from build123d import *

# Parameters (mm, degrees)
SKETCH1_W           = 800
SKETCH1_H           = 650
BOSS_EXTRUDE1_DEPTH = 200
SKETCH2_W           = 796
SKETCH2_H           = 646
CUT_EXTRUDE1_DEPTH  = 198
CUT_EXTRUDE3_REACH  = 802
SKETCH4_R           = 30


with BuildPart() as part:
    # Sketch1 → Boss-Extrude1 (new body)
    with BuildSketch(Plane(origin=(0, 0, 0), x_dir=(1, 0, 0), z_dir=(0, 1, 0))):
        with Locations((400, 325)):
            Rectangle(SKETCH1_W, SKETCH1_H)
    extrude(amount=BOSS_EXTRUDE1_DEPTH)

    # Sketch2 → Cut-Extrude1 (cut)
    with BuildSketch(Plane(origin=(0, 200, 0), x_dir=(1, 0, 0), z_dir=(0, 1, 0))):
        with Locations((400, 325)):
            Rectangle(SKETCH2_W, SKETCH2_H)
    extrude(amount=-CUT_EXTRUDE1_DEPTH, mode=Mode.SUBTRACT)

    # Sketch4 → Cut-Extrude3 (cut, up to next)
    with BuildSketch(Plane(origin=(800, 0, 0), x_dir=(0, 0, -1), z_dir=(1, 0, 0)), mode=Mode.PRIVATE) as cut_extrude3_sk1:
        with Locations((325, 40)):
            Circle(SKETCH4_R)
    cut_extrude3_tool1 = extrude(cut_extrude3_sk1.sketch, amount=-CUT_EXTRUDE3_REACH, mode=Mode.PRIVATE) & part.part
    add(cut_extrude3_tool1.solids().sort_by_distance((800, 40, -325))[0], mode=Mode.SUBTRACT)


solid = part.part
Verification items for the finished model (mm, model axes). A direction names the side the tool comes from. Give positions to 0.01 mm unless a question says otherwise; leave off trailing zeros. Order: outer loops, then holes, each group sorted by start corner. A loop starts at its lowest first (then second) coordinate and runs counter-clockwise, first axis right, second up. Notation, with made-up numbers: M 2.5,84.5 L 52.5,84.5 A23 cw 52.5,112.5 Z; hole C 13.5,-39 d10. An arc over 180 degrees is marked long. Use one line per item in the form item = value. Start each with the question number.
Q1. Scan lines: line 1 along Z through (x, y) = (521.5, 53); line 2 along Y through (x, z) = (799.3, -325); line 3 along X through (y, z) = (33.5, -289). Record each from-to range of solid material in increasing order. Write a range as [from, to].
Q2. Section check C-C (x = 444). Enter the section's corners in (y, z), then the cut area to 3 significant figures.
Q3. Section check B-B (z = -325). Enter the section's corners in (x, y), then the cut area to 3 significant figures.
Q4. Go/stop test with a flat-tipped pin: pin 1 Ø8 at (x, z) = (439.5, -473.5) entering from +Y. Record where the tip stops, or that it passes through.
Q5. Mould release check, pull along X, two halves, no side actions. Record for faces 1 (the flat face through (394, 102, -648)), 2 (the flat face through (0, 99, -320)), 3 (the cylindrical face through (799.01, 41.32, -295.03)), 4 (the flat face through (800, 99, -320)): +X half, -X half, draft (parallel to the pull), parting line (faces both ways), or undercut.
Q6. Section check A-A (y = 188). Enter the section's corners in (x, z).
Q7. Section check D-D (y = 40). Enter the section's corners in (x, z), then the cut area to 3 significant figures.
Q8. Access from +Z, -Z, +X, -X, +Y, -Y to the whole of each face (thin tool, end or side, straight path). Record for faces 5 (the flat face through (394, 0, -330)), 6 (the flat face through (394, 2, -330)).
Evaluation:
q1.line_1 = [-650, -648], [-2, 0]
q1.line_2 = [0, 10], [70, 200]
q1.line_3 = [0, 2], [798, 800]
q2.outline = M 0,-650 L 200,-650 L 200,-648 L 2,-648 L 2,-2 L 200,-2 L 200,0 L 0,0 Z
q2.area = 2,090 mm2
q3.outline = M 0,0 L 800,0 L 800,10 L 798,10 L 798,2 L 2,2 L 2,200 L 0,200 Z; M 798,70 L 800,70 L 800,200 L 798,200 Z
q3.area = 2,270 mm2
q4.pin_1 = 2
q5.face_1 = undercut
q5.face_2 = -X half
q5.face_3 = draft
q5.face_4 = +X half
q6.outline = M 0,-650 L 800,-650 L 800,0 L 0,0 Z; hole M 2,-648 L 798,-648 L 798,-2 L 2,-2 Z
q7.outline = M 0,-650 L 800,-650 L 800,-355 L 798,-355 L 798,-648 L 2,-648 L 2,-2 L 798,-2 L 798,-295 L 800,-295 L 800,0 L 0,0 Z
q7.area = 5,660 mm2
q8.face_5 = +Z, -Z, +X, -X, -Y
q8.face_6 = +Y
